Build history of the part. All positions in model axes, mm. A direction names the side the tool comes from. Round coordinates to 2 decimals unless told otherwise and drop trailing zeros. Write each loop counter-clockwise with the first axis right and the second up, starting at its lowest first coordinate (ties: lowest second). Pieces come first, ordered by that corner, then holes. Notation, with made-up numbers: M 35.5,60 L 89.5,60 A5 cw 89.5,67 Z; hole C -20.75,15.25 d4. An arc over 180 degrees is marked long. Use a Markdown table: item, result.
from build123d import *

# Parameters (mm, degrees)
BOSS_EXTRUDE1_DEPTH     = 10
CUT_EXTRUDE1_DEPTH      = 72.414284285
CUT_EXTRUDE1_DEPTH_BACK = 72.414284285
SKETCH2_R               = 1.5
SKETCH9_W               = 10
SKETCH9_H               = 50
BOSS_EXTRUDE9_DEPTH     = 5
SKETCH10_W              = 10
SKETCH10_H              = 50
BOSS_EXTRUDE10_DEPTH    = 5
BOSS_EXTRUDE11_DEPTH    = 2
SKETCH12_W              = 10
SKETCH12_H              = 10
BOSS_EXTRUDE12_DEPTH    = 5
CUT_EXTRUDE2_START      = 7
SKETCH13_R              = 1.5
CUT_EXTRUDE2_DEPTH      = 7
BOSS_EXTRUDE13_DEPTH    = 2
SKETCH15_W              = 9.981523119
SKETCH15_H              = 10
BOSS_EXTRUDE14_DEPTH    = 30
SKETCH16_R              = 1.5
CUT_EXTRUDE3_DEPTH      = 32
SKETCH17_W              = 10
SKETCH17_H              = 89
BOSS_EXTRUDE15_DEPTH    = 30
SKETCH19_W              = 5
SKETCH19_H              = 89
BOSS_EXTRUDE16_DEPTH    = 15
FILLET1_R               = 5
SKETCH20_R              = 2
CUT_EXTRUDE4_DEPTH      = 149.657324071
SKETCH21_R              = 2
CUT_EXTRUDE5_DEPTH      = 10


with BuildPart() as part:
    # Sketch1 → Boss-Extrude1 (new body)
    with BuildSketch(Plane.XY):
        with BuildLine():
            Line((45.018476881, -25), (50, -25))
            Line((50, -25), (50, 25))
            Line((50, 25), (45, 25))
            ThreePointArc((45, 25), (0, 8), (-45, 25))
            Line((-45, 25), (-50, 25))
            Line((-50, 25), (-50, -25))
            Line((-50, -25), (-45.018476881, -25))
            ThreePointArc((-45.018476881, -25), (0, -8), (45.018476881, -25))
        make_face()
    extrude(amount=BOSS_EXTRUDE1_DEPTH)

    # Sketch2 → Cut-Extrude1 (cut, two sides: drawn at the far end of the back side and taken through both)
    with BuildSketch(Plane(origin=(0, 25, 0), x_dir=(1, 0, 0), z_dir=(0, 1, 0)).offset(-CUT_EXTRUDE1_DEPTH_BACK)):
        with Locations(Location((-48, -5, 0), (0, 0, 180))):
            Circle(SKETCH2_R)
        with Locations(Location((48, -5, 0), (0, 0, 180))):
            Circle(SKETCH2_R)
    extrude(amount=CUT_EXTRUDE1_DEPTH + CUT_EXTRUDE1_DEPTH_BACK, mode=Mode.SUBTRACT)

    # Sketch9 → Boss-Extrude9 (add)
    with BuildSketch(Plane(origin=(50, 0, 0), x_dir=(0, 0, -1), z_dir=(1, 0, 0))):
        with Locations((-5, 0)):
            Rectangle(SKETCH9_W, SKETCH9_H)
    extrude(amount=BOSS_EXTRUDE9_DEPTH)

    # Sketch10 → Boss-Extrude10 (add)
    with BuildSketch(Plane.ZY.offset(50)):
        with Locations((5, 0)):
            Rectangle(SKETCH10_W, SKETCH10_H)
    extrude(amount=BOSS_EXTRUDE10_DEPTH)

    # Sketch11 → Boss-Extrude11 (add)
    with BuildSketch(Plane(origin=(0, 25, 0), x_dir=(1, 0, 0), z_dir=(0, 1, 0))):
        Polygon((50, 0), (50, -7), (45, -7), (45, -10), (55, -10), (55, 0), align=None)
        Polygon((-50, 0), (-50, -7), (-45, -7), (-45, -10), (-55, -10), (-55, 0), align=None)
    extrude(amount=BOSS_EXTRUDE11_DEPTH)

    # Sketch12 → Boss-Extrude12 (add)
    with BuildSketch(Plane(origin=(0, 27, 0), x_dir=(1, 0, 0), z_dir=(0, 1, 0))):
        with Locations((50, -5)):
            Rectangle(SKETCH12_W, SKETCH12_H)
        with Locations((-50, -5)):
            Rectangle(SKETCH12_W, SKETCH12_H)
    extrude(amount=BOSS_EXTRUDE12_DEPTH)

    # Sketch13 → Cut-Extrude2 (cut)
    with BuildSketch(Plane(origin=(0, 25, 0), x_dir=(1, 0, 0), z_dir=(0, 1, 0)).offset(CUT_EXTRUDE2_START)):
        with Locations(Location((48, -5, 0), (0, 0, 180))):
            Circle(SKETCH13_R)
        with Locations(Location((-48, -5, 0), (0, 0, 180))):
            Circle(SKETCH13_R)
    extrude(amount=-CUT_EXTRUDE2_DEPTH, mode=Mode.SUBTRACT)

    # Sketch14 → Boss-Extrude13 (add)
    with BuildSketch(Plane.XZ.offset(25)):
        Polygon((50.009238441, 0), (50.009238441, 7), (45.018476881, 7), (45.018476881, 10), (55, 10), (55, 0), align=None)
        Polygon((-50.009238441, 0), (-50.009238441, 7), (-45.018476881, 7), (-45.018476881, 10), (-55, 10), (-55, 0), align=None)
    extrude(amount=BOSS_EXTRUDE13_DEPTH)

    # Sketch15 → Boss-Extrude14 (add)
    with BuildSketch(Plane.XZ.offset(27)):
        with Locations((-50.00923844, 5)):
            Rectangle(SKETCH15_W, SKETCH15_H)
        with Locations((50.00923844, 5)):
            Rectangle(SKETCH15_W, SKETCH15_H)
    extrude(amount=BOSS_EXTRUDE14_DEPTH)

    # Sketch16 → Cut-Extrude3 (cut)
    with BuildSketch(Plane.XZ.offset(25)):
        with Locations(Location((48, 5, 0), (0, 0, 180))):
            Circle(SKETCH16_R)
        with Locations(Location((-48, 5, 0), (0, 0, 180))):
            Circle(SKETCH16_R)
    extrude(amount=CUT_EXTRUDE3_DEPTH, mode=Mode.SUBTRACT)

    # Sketch17 → Boss-Extrude15 (add)
    with BuildSketch(Plane.ZY.offset(55)):
        with Locations((5, -12.5)):
            Rectangle(SKETCH17_W, SKETCH17_H)
    extrude(amount=BOSS_EXTRUDE15_DEPTH)

    # Sketch19 → Boss-Extrude16 (add)
    with BuildSketch(Plane.XY.offset(10)):
        with Locations((-82.5, -12.5)):
            Rectangle(SKETCH19_W, SKETCH19_H)
    extrude(amount=BOSS_EXTRUDE16_DEPTH)

    # Fillet1
    fillet1_edges = [part.edges().sort_by_distance(p)[0] for p in [
        (-80, -12.5, 10),
    ]]
    fillet(fillet1_edges, radius=FILLET1_R)

    # Sketch20 → Cut-Extrude4 (cut, through all)
    with BuildSketch(Plane(origin=(-80, 0, 0), x_dir=(0, 0, -1), z_dir=(1, 0, 0))):
        with Locations(Location((-20, 9.75, 0), (0, 0, 90))):
            Circle(SKETCH20_R)
        with Locations(Location((-20, -12.5, 0), (0, 0, 90))):
            Circle(SKETCH20_R)
        with Locations(Location((-20, -34.75, 0), (0, 0, 90))):
            Circle(SKETCH20_R)
    extrude(amount=-CUT_EXTRUDE4_DEPTH, mode=Mode.SUBTRACT)

    # Sketch21 → Cut-Extrude5 (cut)
    with BuildSketch(Plane.XY.offset(10)):
        with Locations((-65, 20.875)):
            Circle(SKETCH21_R)
        with Locations((-65, -1.375)):
            Circle(SKETCH21_R)
        with Locations((-65, -23.625)):
            Circle(SKETCH21_R)
        with Locations((-65, -45.875)):
            Circle(SKETCH21_R)
    extrude(amount=-CUT_EXTRUDE5_DEPTH, mode=Mode.SUBTRACT)


solid = part.part
Q1. Cut at D-D on y = -34.75. Give the cut face in (x, z), and give its area (3 significant figures).
Response values:
| item | result |
|---|---|
| outline | M -85,0 L -45.02,0 L -45.02,10 L -75,10 A5 cw -80,15 L -80,18 L -85,18 Z; M -85,22 L -80,22 L -80,25 L -85,25 Z; M 45.02,0 L 55,0 L 55,10 L 45.02,10 Z; hole C -48,5 d3; hole C 48,5 d3 |
| area | 546 mm2 |
Q2. Cut at A-A on y = -12.5. Give the cut face in (x, z), and give its area (3 significant figures).
Response values:
| item | result |
|---|---|
| outline | M -85,0 L -24.35,0 L -24.35,10 L -75,10 A5 cw -80,15 L -80,18 L -85,18 Z; M -85,22 L -80,22 L -80,25 L -85,25 Z; M 24.35,0 L 55,0 L 55,10 L 24.35,10 Z; hole C -48,5 d3; hole C 48,5 d3 |
| area | 959 mm2 |
Q3. Cut at C-C on x = -48. Give the cut face in (y, z).
Response values:
| item | result |
|---|---|
| outline | M -57,0 L -27,0 L -27,3.5 L -57,3.5 Z; M -57,6.5 L -27,6.5 L -27,7 L -25,7 L -25,6.5 L 25,6.5 L 25,7 L 27,7 L 27,6.5 L 32,6.5 L 32,10 L -57,10 Z; M -25,0 L 25,0 L 25,3.5 L -25,3.5 Z; M 27,0 L 32,0 L 32,3.5 L 27,3.5 Z |
Q4. Which spindle directions (+Z, -Z, +X, -X, +Y, -Y) get a long thin tool onto all of the face, cutting with end or side? Do faces 4 (the cylindrical face through (-82.465, -12.76, 21.983)), 5 (the flat face through (47, 25, 3)), 6 (the cylindrical face through (-65.43, -47.83, 5.07)), 7 (the flat face through (45.018, -41, 5)), 8 (the flat face through (-45, 29, 5)). Say none if no direction does.
Response values:
| item | result |
|---|---|
| face 4 | +X, -X |
| face 5 | -Z |
| face 6 | +Z, -Z |
| face 7 | +Z, -Z, -Y |
| face 8 | +Z, -Z, +Y |
Q5. Drop flat-ended pins along their axis: P1, Ø4, axis at x = -47.5, y = -15, coming from the +Z side; P2, Ø10, axis at x = -13.5, z = 9.5, coming from the +Y side; P3, Ø10, axis at y = 11.5, z = 20, coming from the +X side; P4, Ø2.5, axis at x = 48, z = 5, coming from the -Y side. Give the stop position or say it passes through.
Response values:
| item | result |
|---|---|
| P1 | stops at z = 10 |
| P2 | stops at y = 10.56 |
| P3 | stops at x = -80 |
| P4 | passes through |
Q6. Drill centre lines: L1, parallel to X at y = -50, z = 5; L2, parallel to Y at x = -65, z = 5 (3 decimals); L3, parallel to Y at x = 45.5, z = 4. Where is each one in solid material? Low to high.
Response values:
| item | result |
|---|---|
| L1 | x = -85 to -49.5, -46.5 to -45.02, 45.02 to 46.5, 49.5 to 55 |
| L2 | y = -57 to -47.875, -43.875 to -25.625, -21.625 to -3.375, 0.625 to 18.875, 22.875 to 32 |
| L3 | y = -57 to -27, -25 to 25, 27 to 32 |
Q7. Cut at B-B on x = -65. Give the cut face in (y, z) (3 decimals).
Response values:
| item | result |
|---|---|
| outline | M -57,0 L -47.875,0 L -47.875,10 L -57,10 Z; M -43.875,0 L -25.625,0 L -25.625,10 L -43.875,10 Z; M -21.625,0 L -3.375,0 L -3.375,10 L -21.625,10 Z; M 0.625,0 L 18.875,0 L 18.875,10 L 0.625,10 Z; M 22.875,0 L 32,0 L 32,10 L 22.875,10 Z |
Q8. Two-plate mould, pull along Z, no slides. Class faces 1 (the cylindrical face through (-66.5, 22.2, 5.1)), 2 (the cylindrical face through (49.5, -0.35, 5.07)), 3 (the cylindrical face through (-78, -12, 11)): +Z half, -Z half, draft (parallel to the pull), parting line (faces both ways), or undercut.
Response values:
| item | result |
|---|---|
| face 1 | draft |
| face 2 | undercut |
| face 3 | +Z half |
